The model under review builds one solid part; all positions refer to its coordinate system, in mm. Face numbers are marked on the shaded views. A direction names the side the tool comes from. Round coordinates to 2 decimals unless told otherwise and drop trailing zeros. Write each loop counter-clockwise with the first axis right and the second up, starting at its lowest first coordinate (ties: lowest second). Pieces come first, ordered by that corner, then holes. Notation, with made-up numbers: (6, 2) - (52, 2) arc R23 cw to (52, 39) - close; hole circle Ø8 at (72.25, 4). An arc over 180 degrees is marked (long way). Use one line per item in the form item = value.
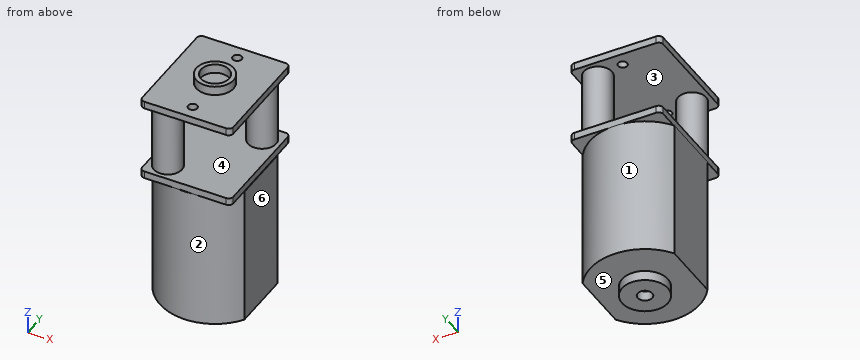
from build123d import *

# Parameters (mm, degrees)
EXTRUDE_1_DEPTH     = 15.4
SKETCH_2_R          = 2.52
SKETCH_2_R_2        = 0.8
EXTRUDE_2_DEPTH     = 1.1
SKETCH_5_W          = 10
SKETCH_5_H          = 12
EXTRUDE_3_DEPTH     = 0.8
SKETCH_7_R          = 1.55
EXTRUDE_4_DEPTH     = 7.6
SKETCH_8_W          = 10
SKETCH_8_H          = 12
EXTRUDE_5_DEPTH     = 0.8
SKETCH_9_R          = 2.05
SKETCH_9_R_2        = 1.55
EXTRUDE_6_DEPTH     = 1
FILLET_1_R          = 0.5
CUT_EXTRUDE_1_REACH = 28.881
SKETCH_10_R         = 0.5


with BuildPart() as part:
    # Эскиз1 → Бобышка-Вытянуть1 (new body)
    with BuildSketch(Plane.XY):
        with BuildLine():
            Line((5.05, -3.33166625), (5.05, 3.33166625))
            ThreePointArc((5.05, 3.33166625), (0, 6.05), (-5.05, 3.33166625))
            Line((-5.05, 3.33166625), (-5.05, -3.33166625))
            ThreePointArc((-5.05, -3.33166625), (0, -6.05), (5.05, -3.33166625))
        make_face()
    extrude(amount=EXTRUDE_1_DEPTH)

    # Эскиз2 → Бобышка-Вытянуть2 (add)
    with BuildSketch(Plane(origin=(0, 0, 0), x_dir=(-1, 0, 0), z_dir=(0, 0, -1))):
        Circle(SKETCH_2_R)
        Circle(SKETCH_2_R_2, mode=Mode.SUBTRACT)
    extrude(amount=EXTRUDE_2_DEPTH)

    # Эскиз5 → Бобышка-Вытянуть3 (add)
    with BuildSketch(Plane.XY.offset(15.4)):
        Rectangle(SKETCH_5_W, SKETCH_5_H)
    extrude(amount=EXTRUDE_3_DEPTH)

    # Эскиз7 → Бобышка-Вытянуть4 (add)
    with BuildSketch(Plane.XY.offset(16.2)):
        with Locations(Location((3, 4, 0), (0, 0, 180))):
            Circle(SKETCH_7_R)
        with Locations(Location((-3, -4, 0), (0, 0, 180))):
            Circle(SKETCH_7_R)
    extrude(amount=EXTRUDE_4_DEPTH)

    # Эскиз8 → Бобышка-Вытянуть5 (add)
    with BuildSketch(Plane.XY.offset(23.8)):
        Rectangle(SKETCH_8_W, SKETCH_8_H)
    extrude(amount=EXTRUDE_5_DEPTH)

    # Эскиз9 → Бобышка-Вытянуть6 (add)
    with BuildSketch(Plane.XY.offset(24.6)):
        Circle(SKETCH_9_R)
        Circle(SKETCH_9_R_2, mode=Mode.SUBTRACT)
    extrude(amount=EXTRUDE_6_DEPTH)

    # Скругление1
    fillet_1_edges = [part.edges().sort_by_distance(p)[0] for p in [
        (-5, 6, 15.8),
        (-5, -6, 15.8),
        (5, -6, 15.8),
        (5, 6, 15.8),
        (5, 6, 24.2),
        (-5, 6, 24.2),
        (-5, -6, 24.2),
        (5, -6, 24.2),
    ]]
    fillet(fillet_1_edges, radius=FILLET_1_R)

    # Эскиз10 → Вырез-Вытянуть1 (cut, up to next)
    with BuildSketch(Plane.XY.offset(24.6), mode=Mode.PRIVATE) as cut_extrude_1_sk1:
        with Locations((0, -4.5)):
            Circle(SKETCH_10_R)
    cut_extrude_1_tool1 = extrude(cut_extrude_1_sk1.sketch, amount=-CUT_EXTRUDE_1_REACH, mode=Mode.PRIVATE) & part.part
    # Эскиз10 → Вырез-Вытянуть1 (cut, up to next)
    with BuildSketch(Plane.XY.offset(24.6), mode=Mode.PRIVATE) as cut_extrude_1_sk2:
        with Locations((0, 4.5)):
            Circle(SKETCH_10_R)
    cut_extrude_1_tool2 = extrude(cut_extrude_1_sk2.sketch, amount=-CUT_EXTRUDE_1_REACH, mode=Mode.PRIVATE) & part.part
    add(cut_extrude_1_tool1.solids().sort_by_distance((0, -4.5, 24.6))[0], mode=Mode.SUBTRACT)
    add(cut_extrude_1_tool2.solids().sort_by_distance((0, 4.5, 24.6))[0], mode=Mode.SUBTRACT)


solid = part.part
(1) To check wall thickness, follow L1, parallel to Y at x = 0, z = 24; L2, parallel to Y at x = 0, z = 25.25; L3, parallel to Z at x = 0.5, y = 3.5. State the ranges of each line that lie inside material, in increasing order.
Geometry results:
L1 = -6 to -5, -4 to 4, 5 to 6
L2 = -2.05 to -1.55, 1.55 to 2.05
L3 = 0 to 16.2, 23.8 to 24.6
(2) Machinability: for the marked faces 1, 2 and 3, which of the approach directions +Z, -Z, +X, -X, +Y, -Y give a long, thin tool a straight path to every point of the face, cutting with its end or side? Answer none if there is none.
Geometry results:
face_1 = -Z, +Y
face_2 = -Z, -Y
face_3 = none
(3) Add section B-B on z = 18.75. Write out the cut boundary in (x, y), then the cut area to 3 significant figures.
Geometry results:
outline = circle Ø3.1 at (-3, -4); circle Ø3.1 at (3, 4)
area = 15.1 mm2
(4) Insertion check: P1, Ø0.9, axis at x = -1, z = 24.5, coming from the +Y side; P2, Ø1.4, axis at x = 0, y = 0, coming from the +Z side; P3, Ø0.8, axis at x = -3, y = 4, coming from the -Z side. Each pin has a flat end and moves straight along its axis. Give the tip position at first contact, or say it passes through.
Geometry results:
P1 = 6
P2 = 24.6
P3 = 0
(5) The part is to be moulded in two halves that separate along Z. For the marked faces 4, 5 and 6, say which applies: +Z half, -Z half, draft (parallel to the pull), parting line (faces both ways), or undercut.
Geometry results:
face_4 = undercut
face_5 = -Z half
face_6 = draft
(6) Add section D-D on y = 5.25. Write out the cut boundary in (x, z), then the cut area to 3 significant figures.
Geometry results:
outline = (-5, 15.4) - (-3.01, 15.4) - (-3.01, 0) - (3.01, 0) - (3.01, 15.4) - (5, 15.4) - (5, 16.2) - (3.92, 16.2) - (3.92, 23.8) - (5, 23.8) - (5, 24.6) - (-5, 24.6) - (-5, 23.8) - (2.08, 23.8) - (2.08, 16.2) - (-5, 16.2) - close
area = 123 mm2
(7) Add section C-C on x = -3.5. Write out the cut boundary in (y, z).
Geometry results:
outline = (-6, 15.4) - (-4.93, 15.4) - (-4.93, 0) - (4.93, 0) - (4.93, 15.4) - (6, 15.4) - (6, 16.2) - (-2.53, 16.2) - (-2.53, 23.8) - (6, 23.8) - (6, 24.6) - (-6, 24.6) - (-6, 23.8) - (-5.47, 23.8) - (-5.47, 16.2) - (-6, 16.2) - close
(8) Add section A-A on y = 0. Write out the cut boundary in (x, z).
Geometry results:
outline = (-5.05, 0) - (-2.52, 0) - (-2.52, -1.1) - (-0.8, -1.1) - (-0.8, 0) - (0.8, 0) - (0.8, -1.1) - (2.52, -1.1) - (2.52, 0) - (5.05, 0) - (5.05, 15.4) - (5, 15.4) - (5, 16.2) - (-5, 16.2) - (-5, 15.4) - (-5.05, 15.4) - close; (-5, 23.8) - (5, 23.8) - (5, 24.6) - (2.05, 24.6) - (2.05, 25.6) - (1.55, 25.6) - (1.55, 24.6) - (-1.55, 24.6) - (-1.55, 25.6) - (-2.05, 25.6) - (-2.05, 24.6) - (-5, 24.6) - close
